For this review, take the finished solid that the model builds, in its own axes (mm). A direction names the side the tool comes from. Round coordinates to 2 decimals unless told otherwise and drop trailing zeros. Write each loop counter-clockwise with the first axis right and the second up, starting at its lowest first coordinate (ties: lowest second). Pieces come first, ordered by that corner, then holes. Notation, with made-up numbers: (14.25, 51.25) -> (22.25, 51.25) arc R20 ccw to (22.25, 67.25) -> close; hole circle Ø4 at (12, 26). An arc over 180 degrees is marked (long way). Answer in a Markdown table with one row per item.
from build123d import *

# Parameters (mm, degrees)
SKETCH1_W           = 482.6
SKETCH1_H           = 304.8
BOSS_EXTRUDE1_DEPTH = 26.416
CUT_EXTRUDE3_DEPTH  = 3.175
SKETCH3_R           = 6.35
CUT_EXTRUDE2_DEPTH  = 27.416


with BuildPart() as part:
    # Sketch1 → Boss-Extrude1 (new body)
    with BuildSketch(Plane(origin=(0, 0, 0), x_dir=(1, 0, 0), z_dir=(0, 1, 0))):
        Rectangle(SKETCH1_W, SKETCH1_H)
    extrude(amount=BOSS_EXTRUDE1_DEPTH)

    # Sketch2 → Cut-Extrude3 (cut)
    with BuildSketch(Plane(origin=(0, 26.416, 0), x_dir=(1, 0, 0), z_dir=(0, 1, 0))):
        with BuildLine():
            Line((-70.7865, 120.142), (-70.7865, -120.142))
            ThreePointArc((-70.7865, -120.142), (-64.4365, -113.792), (-58.0865, -120.142))
            Line((-58.0865, -120.142), (-58.0865, 120.142))
            ThreePointArc((-58.0865, 120.142), (-64.4365, 113.792), (-70.7865, 120.142))
        make_face()
        with BuildLine():
            ThreePointArc((-58.0865, 120.142), (-64.4365, 126.492), (-70.7865, 120.142))
            Line((-70.7865, 120.142), (-58.0865, 120.142))
        make_face()
        with BuildLine():
            Line((-58.0865, 120.142), (-70.7865, 120.142))
            ThreePointArc((-70.7865, 120.142), (-64.4365, 113.792), (-58.0865, 120.142))
        make_face()
        with BuildLine():
            ThreePointArc((-58.0865, -120.142), (-64.4365, -113.792), (-70.7865, -120.142))
            Line((-70.7865, -120.142), (-58.0865, -120.142))
        make_face()
        with BuildLine():
            Line((-58.0865, -120.142), (-70.7865, -120.142))
            ThreePointArc((-70.7865, -120.142), (-64.4365, -126.492), (-58.0865, -120.142))
        make_face()
        with BuildLine():
            ThreePointArc((58.0865, 120.142), (64.4365, 113.792), (70.7865, 120.142))
            Line((70.7865, 120.142), (58.0865, 120.142))
        make_face()
        with BuildLine():
            Line((58.0865, 120.142), (70.7865, 120.142))
            ThreePointArc((70.7865, 120.142), (64.4365, 126.492), (58.0865, 120.142))
        make_face()
        with BuildLine():
            Line((70.7865, -120.142), (70.7865, 120.142))
            ThreePointArc((70.7865, 120.142), (64.4365, 113.792), (58.0865, 120.142))
            Line((58.0865, 120.142), (58.0865, -120.142))
            ThreePointArc((58.0865, -120.142), (64.4365, -113.792), (70.7865, -120.142))
        make_face()
        with BuildLine():
            ThreePointArc((58.0865, -120.142), (64.4365, -126.492), (70.7865, -120.142))
            Line((70.7865, -120.142), (58.0865, -120.142))
        make_face()
        with BuildLine():
            Line((58.0865, -120.142), (70.7865, -120.142))
            ThreePointArc((70.7865, -120.142), (64.4365, -113.792), (58.0865, -120.142))
        make_face()
    extrude(amount=-CUT_EXTRUDE3_DEPTH, mode=Mode.SUBTRACT)

    # Sketch3 → Cut-Extrude2 (cut, through all)
    with BuildSketch(Plane(origin=(0, 26.416, 0), x_dir=(1, 0, 0), z_dir=(0, 1, 0))):
        with Locations((-185.0865, -80.01)):
            Circle(SKETCH3_R)
        with Locations((-159.6865, -80.01)):
            Circle(SKETCH3_R)
        with Locations((-159.6865, 80.01)):
            Circle(SKETCH3_R)
        with Locations((-185.0865, 80.01)):
            Circle(SKETCH3_R)
        with Locations((159.6865, -80.01)):
            Circle(SKETCH3_R)
        with Locations((185.0865, -80.01)):
            Circle(SKETCH3_R)
        with Locations((159.6865, 80.01)):
            Circle(SKETCH3_R)
        with Locations((185.0865, 80.01)):
            Circle(SKETCH3_R)
    extrude(amount=-CUT_EXTRUDE2_DEPTH, mode=Mode.SUBTRACT)


solid = part.part
1) For faces 1 (the flat face through (-65, 23.241, -2)), 2 (the flat face through (-241.3, 13, 2)), list the 3-axis set-ups (+Z, -Z, +X, -X, +Y, -Y) from which the entire face can be reached by the end or side of a thin tool; tool diameter is ignored.
Solved:
| item | result |
|---|---|
| face 1 | +Y |
| face 2 | +Z, -Z, -X, +Y, -Y |
2) Clearance check with flat-ended pins moving along their axes: pin 1 Ø10 at (x, z) = (185.09, -80.01) entering from +Y; pin 2 Ø6.5 at (x, z) = (65.5, 24.5) entering from +Y. State where each tip first meets the part, or that it passes through.
Solved:
| item | result |
|---|---|
| pin 1 | through |
| pin 2 | y = 23.24 |
3) Consider section A-A on z = 80.01. State the section outline as (x, y) points, then the cut area to 3 significant figures.
Solved:
| item | result |
|---|---|
| outline | (-241.3, 0) -> (-191.44, 0) -> (-191.44, 26.42) -> (-241.3, 26.42) -> close; (-178.74, 0) -> (-166.04, 0) -> (-166.04, 26.42) -> (-178.74, 26.42) -> close; (-153.34, 0) -> (153.34, 0) -> (153.34, 26.42) -> (70.79, 26.42) -> (70.79, 23.24) -> (58.09, 23.24) -> (58.09, 26.42) -> (-58.09, 26.42) -> (-58.09, 23.24) -> (-70.79, 23.24) -> (-70.79, 26.42) -> (-153.34, 26.42) -> close; (166.04, 0) -> (178.74, 0) -> (178.74, 26.42) -> (166.04, 26.42) -> close; (191.44, 0) -> (241.3, 0) -> (241.3, 26.42) -> (191.44, 26.42) -> close |
| area | 11,300 mm² |
4) For line 1 (X direction, y = 13.25, z = 80.01); line 2 (Z direction, x = -189, y = 20); line 3 (Y direction, x = -61.5, z = 85), list the stretches that pass through material, from the lowest coordinate up. Write a range as [from, to].
Solved:
| item | result |
|---|---|
| line 1 | [-241.3, -191.44], [-178.74, -166.04], [-153.34, 153.34], [166.04, 178.74], [191.44, 241.3] |
| line 2 | [-152.4, -85.01], [-75.01, 75.01], [85.01, 152.4] |
| line 3 | [0, 23.24] |
5) Mouldability with a two-part tool opening along Z and no side actions: class faces 3 (the cylindrical face through (-153.63, 13.39, 78.1)), 4 (the flat face through (-3, 13, 152.4)), 5 (the flat face through (-3, 13, -152.4)), 6 (the flat face through (241.3, 13, 2)) as pulls with the +Z half, pulls with the -Z half, needs draft (parallel to the pull), parting line crosses it, or undercut.
Solved:
| item | result |
|---|---|
| face 3 | undercut |
| face 4 | pulls with the +Z half |
| face 5 | pulls with the -Z half |
| face 6 | needs draft |
